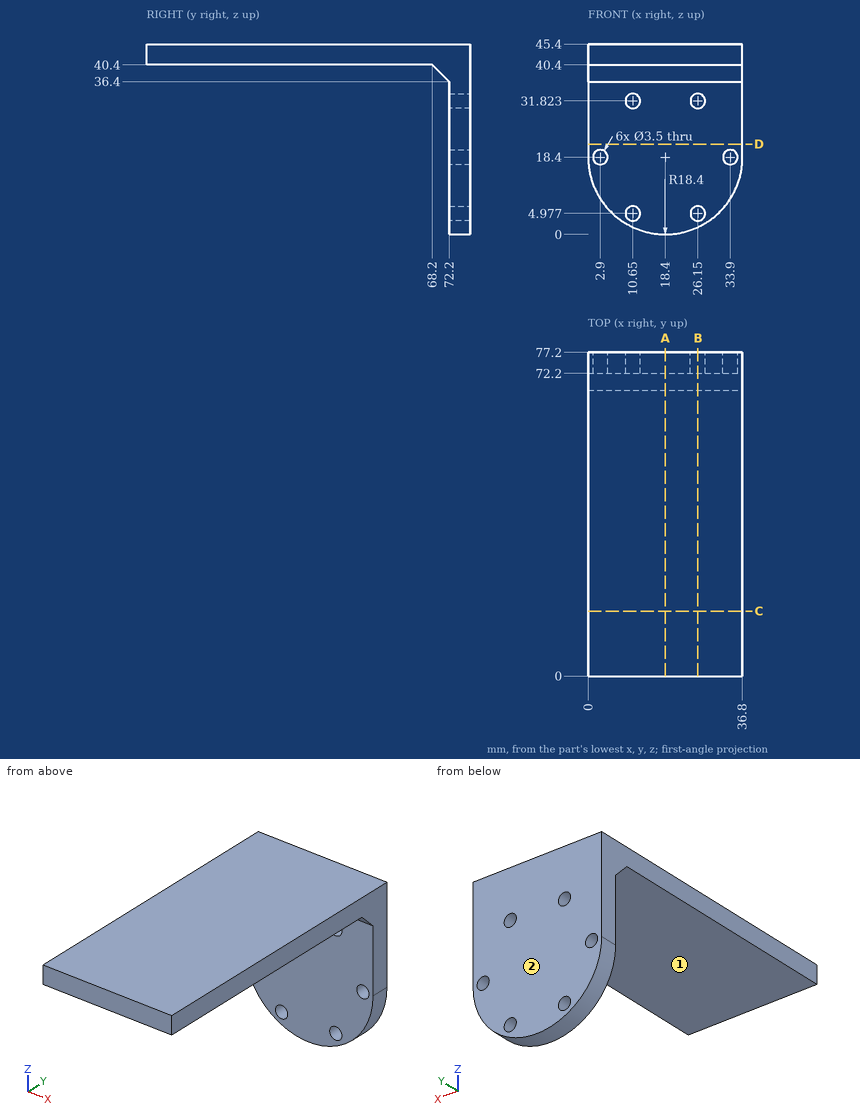
Study the drawing (mm; zero at the part's minimum x, y, z) and answer. A direction names the side the tool comes from. Coordinates: 2 decimals unless noted, no trailing zeros. Loops run counter-clockwise (first coordinate to the right, second up) from the corner with the lowest first, then second, coordinate; pieces in that order, holes last. Notation, with made-up numbers: M 81.5,-26.5 L 103.5,-26.5 A13 cw 103.5,-12.5 Z; hole C -9,-8 d8. An arc over 180 degrees is marked long. Answer in a Markdown table with one row per item. Add a question column.
1. Find section A-A, the plane x = 18.4. Write down the section's boundary in (y, z), then the cut area to 3 significant figures.
2. A tool of negligible diameter and unlimited length cuts with its end or side. For the marked faces 1 and 2, from which of +Z, -Z, +X, -X, +Y, -Y can it reach the whole face along a straight path? Write none if from no direction.
3. Find section B-B, the plane x = 26.15. Write down the section's boundary in (y, z).
4. Find section D-D, the plane z = 21.5. Write down the section's boundary in (x, y), then the cut area to 3 significant figures.
5. Flat-ended cylindrical pins translate along their axes: P1, Ø5.5, axis at x = 10.65, z = 31.82, coming from the -Y side; P2, Ø10, axis at y = 12.5, z = 39.5, coming from the -X side; P3, Ø2, axis at x = 19, y = 48.5, coming from the -Z side. Find the tip coordinate at first contact, or state that the pin passes through.
6. Consider L1, parallel to X at y = 75.3, z = 18.4; L2, parallel to Y at x = 11, z = 9; L3, parallel to Z at x = 10.5, y = 18. Determine where each line is inside the solid, lowest interval first.
7. Find section C-C, the plane y = 15.5. Write down the section's boundary in (x, z).
Reported:
| question | item | result |
|---|---|---|
| 1 | outline | M 0,40.4 L 68.2,40.4 L 72.2,36.4 L 72.2,0 L 77.2,0 L 77.2,45.4 L 0,45.4 Z |
| 1 | area | 596 mm^2 |
| 2 | face 1 | -Z, +X, -X, -Y |
| 2 | face 2 | +Z, -Z, +X, -X, +Y |
| 3 | outline | M 0,40.4 L 68.2,40.4 L 72.2,36.4 L 72.2,33.57 L 77.2,33.57 L 77.2,45.4 L 0,45.4 Z; M 72.2,1.71 L 77.2,1.71 L 77.2,3.23 L 72.2,3.23 Z; M 72.2,6.73 L 77.2,6.73 L 77.2,30.07 L 72.2,30.07 Z |
| 4 | outline | M 0,72.2 L 36.8,72.2 L 36.8,77.2 L 0,77.2 Z |
| 4 | area | 184 mm^2 |
| 5 | P1 | stops at y = 72.2 |
| 5 | P2 | stops at x = 0 |
| 5 | P3 | stops at z = 40.4 |
| 6 | L1 | x = 0 to 1.15, 4.65 to 32.15, 35.65 to 36.8 |
| 6 | L2 | y = 72.2 to 77.2 |
| 6 | L3 | z = 40.4 to 45.4 |
| 7 | outline | M 0,40.4 L 36.8,40.4 L 36.8,45.4 L 0,45.4 Z |
